Drawing for the job (mm, zero at the part's lowest x, y, z). A direction names the side the tool comes from. Coordinates: 2 decimals unless noted, no trailing zeros. Order: outer loops, then holes, each group sorted by start corner. A loop starts at its lowest first (then second) coordinate and runs counter-clockwise, first axis right, second up.
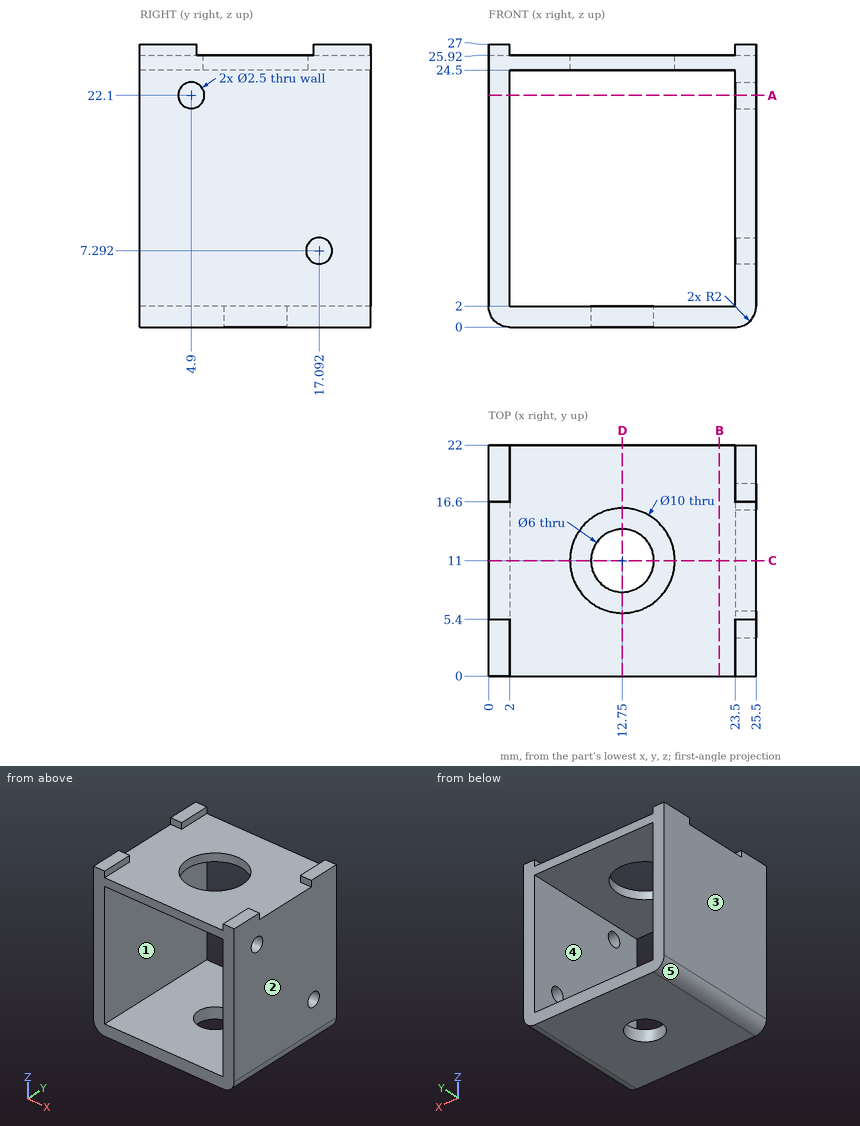
(1) Drop a flat-ended pin along its axis: pin 1 (1.5 mm diameter, centred on x = 15, y = 16.5, fed in from +Z). Give the stop position or say it passes through.
(2) Tool access for the marked faces 1 and 2: list every direction of +Z, -Z, +X, -X, +Y, -Y with a clear straight run to the whole face (end or side of a thin tool).
(3) Slice it at B-B, the plane x = 22. Give the cut face in (y, z).
(4) Slice it at A-A, the plane z = 22.1. Give the cut face in (x, y).
(5) Pull direction Z, two halves, no side cores. Call the marked faces 3, 4 and 5: +Z half, -Z half, draft (parallel to the pull), parting line (faces both ways), or undercut.
(6) Probe line 1 (Y direction, x = 12.75, z = 1.2); line 2 (X direction, y = 17, z = 19.75); line 3 (Z direction, x = 4.25, y = 6). List the from-to ranges inside material, lowest first.
(7) Slice it at D-D, the plane x = 12.75. Give the cut face in (y, z).
(8) Slice it at C-C, the plane y = 11. Give the cut face in (x, z).
Here are the results:
1. pin 1: stops at z = 25.92
2. face 1: +Y, -Y
2. face 2: +Z, -Z, +X, +Y, -Y
3. outline: (0, 0) - (22, 0) - (22, 2) - (0, 2) - close; (0, 24.5) - (22, 24.5) - (22, 25.92) - (0, 25.92) - close
4. outline: (0, 0) - (2, 0) - (2, 22) - (0, 22) - close; (23.5, 0) - (25.5, 0) - (25.5, 3.65) - (23.5, 3.65) - close; (23.5, 6.15) - (25.5, 6.15) - (25.5, 22) - (23.5, 22) - close
5. face 3: draft
5. face 4: undercut
5. face 5: -Z half
6. line 1: y = 0 to 8, 14 to 22
6. line 2: x = 0 to 2, 23.5 to 25.5
6. line 3: z = 0 to 2, 24.5 to 25.92
7. outline: (0, 0) - (8, 0) - (8, 2) - (0, 2) - close; (0, 24.5) - (6, 24.5) - (6, 25.92) - (0, 25.92) - close; (14, 0) - (22, 0) - (22, 2) - (14, 2) - close; (16, 24.5) - (22, 24.5) - (22, 25.92) - (16, 25.92) - close
8. outline: (0, 2) arc R2 ccw to (2, 0) - (9.75, 0) - (9.75, 2) - (2, 2) - (2, 24.5) - (7.75, 24.5) - (7.75, 25.92) - (0, 25.92) - close; (15.75, 0) - (23.5, 0) arc R2 ccw to (25.5, 2) - (25.5, 25.92) - (17.75, 25.92) - (17.75, 24.5) - (23.5, 24.5) - (23.5, 2) - (15.75, 2) - close
